Build history of the part. All positions in model axes, mm. Face numbers are marked on the shaded views. Give positions to 0.01 mm unless a question says otherwise; leave off trailing zeros. Order: outer loops, then holes, each group sorted by start corner. A loop starts at its lowest first (then second) coordinate and runs counter-clockwise, first axis right, second up. Notation, with made-up numbers: (-35.75, -40) -> (20.25, -40) arc R20 cw to (20.25, -4) -> close; hole circle Ø10 at (-28.5, 40.25). An arc over 180 degrees is marked (long way). Use a Markdown table: item, result. Add a question column.
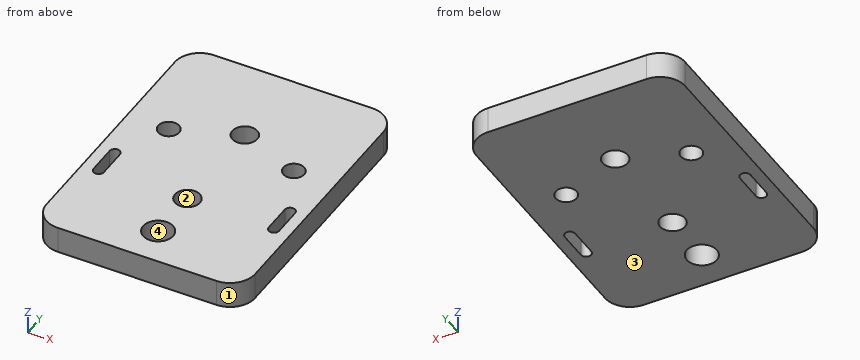
```python
from build123d import *

# Parameters (mm, degrees)
F0_W     = 19.2
F0_H     = 68
F0_R     = 6
F0_R_2   = 3
F0_R_3   = 4.75
F0_R_4   = 3.6
F0_R_5   = 2.51
F0_W_2   = 2.745
F0_H_2   = 7
F1_DEPTH = 6.35


with BuildPart() as f1:
    # F0 (on Top) → F1 (new body)
    with BuildSketch(Plane.XY):
        Rectangle(F0_W, F0_H)
        with Locations((0, -24.8)):
            Circle(F0_R, mode=Mode.SUBTRACT)
        with Locations((0, -12)):
            Circle(F0_R_2, mode=Mode.SUBTRACT)
        with Locations((0, 13)):
            Circle(F0_R_2, mode=Mode.SUBTRACT)
        with BuildLine():
            Line((-25, -5.5), (-22.255, -5.5))
            ThreePointArc((-22.255, -5.5), (-21.005, -4.25), (-19.755, -5.5))
            Line((-19.755, -5.5), (-19.755, -12.5))
            ThreePointArc((-19.755, -12.5), (-21.005, -13.75), (-22.255, -12.5))
            Line((-22.255, -12.5), (-25, -12.5))
            Line((-25, -12.5), (-25, -28))
            ThreePointArc((-25, -28), (-23.242641, -32.242641), (-19, -34))
            Line((-19, -34), (-10, -34))
            Line((-10, -34), (-9.6, -34))
            Line((-9.6, -34), (-9.6, 34))
            Line((-9.6, 34), (-19, 34))
            ThreePointArc((-19, 34), (-23.242641, 32.242641), (-25, 28))
            Line((-25, 28), (-25, -5.5))
        make_face()
        with Locations((-15, 7.1)):
            Circle(F0_R_3, mode=Mode.SUBTRACT)
        with BuildLine():
            Line((19, 34), (9.6, 34))
            Line((9.6, 34), (9.6, -34))
            Line((9.6, -34), (19, -34))
            ThreePointArc((19, -34), (23.242641, -32.242641), (25, -28))
            Line((25, -28), (25, -12.5))
            Line((25, -12.5), (22.255, -12.5))
            ThreePointArc((22.255, -12.5), (21.005, -13.75), (19.755, -12.5))
            Line((19.755, -12.5), (19.755, -5.5))
            ThreePointArc((19.755, -5.5), (21.005, -4.25), (22.255, -5.5))
            Line((22.255, -5.5), (25, -5.5))
            Line((25, -5.5), (25, 28))
            ThreePointArc((25, 28), (23.242641, 32.242641), (19, 34))
        make_face()
        with Locations((15, 7.1)):
            Circle(F0_R_3, mode=Mode.SUBTRACT)
        with Locations((0, -24.8)):
            Circle(F0_R)
        with Locations((0, -24.8)):
            Circle(F0_R_4, mode=Mode.SUBTRACT)
        with Locations((15, 7.1)):
            Circle(F0_R_3)
        with Locations((15, 7.1)):
            Circle(F0_R_5, mode=Mode.SUBTRACT)
        with Locations((-15, 7.1)):
            Circle(F0_R_3)
        with Locations((-15, 7.1)):
            Circle(F0_R_5, mode=Mode.SUBTRACT)
        with Locations((-23.6275, -9)):
            Rectangle(F0_W_2, F0_H_2)
        with Locations((23.6275, -9)):
            Rectangle(F0_W_2, F0_H_2)
    extrude(amount=F1_DEPTH)


solid = f1.part
```
(1) Wall check: probe 1 along Y at (x, z) = (0, 1.5); probe 2 along X at (y, z) = (-8.5, 2.5) (3 decimals); probe 3 along Y at (x, z) = (2.5, 4.25). Give the ranges that are in metal, low to high.
(2) Mould opens along X. For the marked faces 1, 2, 3 and 4 say: released by +X, released by -X, zero draft, split by the parting line, or undercut.
(3) Band-saw the part on A-A on y = -24.8. Give the cut face in (x, z).
(4) Band-saw the part on B-B on x = -15. Give the cut face in (y, z), plus the area to 3 significant figures.
(5) Band-saw the part on D-D on y = 7.1. Give the cut face in (x, z), plus the area to 3 significant figures.
(6) Band-saw the part on C-C on z = 3.75. Give the cut face in (x, y) (3 decimals).
Response:
| question | item | result |
|---|---|---|
| 1 | probe 1 | y = -34 to -28.4, -21.2 to -15, -9 to 10, 16 to 34 |
| 1 | probe 2 | x = -25 to -22.255, -19.755 to 19.755, 22.255 to 25 |
| 1 | probe 3 | y = -34 to -27.39, -22.21 to -13.66, -10.34 to 11.34, 14.66 to 34 |
| 2 | face 1 | released by +X |
| 2 | face 2 | undercut |
| 2 | face 3 | zero draft |
| 2 | face 4 | undercut |
| 3 | outline | (-25, 0) -> (-3.6, 0) -> (-3.6, 6.35) -> (-25, 6.35) -> close; (3.6, 0) -> (25, 0) -> (25, 6.35) -> (3.6, 6.35) -> close |
| 4 | outline | (-34, 0) -> (4.59, 0) -> (4.59, 6.35) -> (-34, 6.35) -> close; (9.61, 0) -> (34, 0) -> (34, 6.35) -> (9.61, 6.35) -> close |
| 4 | area | 400 mm² |
| 5 | outline | (-25, 0) -> (-17.51, 0) -> (-17.51, 6.35) -> (-25, 6.35) -> close; (-12.49, 0) -> (12.49, 0) -> (12.49, 6.35) -> (-12.49, 6.35) -> close; (17.51, 0) -> (25, 0) -> (25, 6.35) -> (17.51, 6.35) -> close |
| 5 | area | 254 mm² |
| 6 | outline | (-25, -28) arc R6 ccw to (-19, -34) -> (19, -34) arc R6 ccw to (25, -28) -> (25, 28) arc R6 ccw to (19, 34) -> (-19, 34) arc R6 ccw to (-25, 28) -> close; hole (-22.255, -12.5) arc R1.25 ccw to (-19.755, -12.5) -> (-19.755, -5.5) arc R1.25 ccw to (-22.255, -5.5) -> close; hole circle Ø5.02 at (-15, 7.1); hole circle Ø7.2 at (0, -24.8); hole circle Ø6 at (0, -12); hole circle Ø6 at (0, 13); hole circle Ø5.02 at (15, 7.1); hole (19.755, -12.5) arc R1.25 ccw to (22.255, -12.5) -> (22.255, -5.5) arc R1.25 ccw to (19.755, -5.5) -> close |
